Work out the finished part from the listing and answer in its coordinate system (mm). A direction names the side the tool comes from. Coordinates: 2 decimals unless noted, no trailing zeros. Write each loop counter-clockwise with the first axis right and the second up, starting at its lowest first coordinate (ties: lowest second). Pieces come first, ordered by that corner, then holes. Notation, with made-up numbers: (21, 17) - (74, 17) arc R18 ccw to (74, 22) - close; hole circle Ø9 at (28, -31). An arc over 180 degrees is marked (long way). Use one line per item in the form item = value. Start each with the question number.
Item 1: A cutting plane is placed at C-C (y = -12). Write down the section's boundary in (x, z).
Item 2: Consider probe 1 along Y at (x, z) = (1.7, 0); probe 2 along Y at (x, z) = (2.75, 0); probe 3 along X at (y, z) = (-44, -5.5). Determine where each line is inside the solid, lowest interval first.
Item 3: For faces 5 (the cylindrical face through (13.557, 11.892, 0.14)), 6 (the flat face through (10, -39, 0)), determine the directions among +Z, -Z, +X, -X, +Y, -Y from which every point of the face is accessible in a straight line to the end or side of a thin tool.
Item 4: A cutting plane is placed at D-D (y = -71). Write down the section's boundary in (x, z), then the cut area to 3 significant figures.
Item 5: A cutting plane is placed at A-A (z = 0). Write down the section's boundary in (x, y), then the cut area to 3 significant figures.
Item 6: Given pin 1 (2.5 mm diameter, centred on x = 12.5, z = 2, fed in from -Y); pin 2 (1 mm diameter, centred on y = -32.5, z = 0.5, fed in from +X), each flat-ended and moving along its own axis, determine where each tip first touches the part or whether it passes through.
Item 7: A cutting plane is placed at B-B (x = 3). Write down the section's boundary in (y, z), then the cut area to 3 significant figures.
Item 8: Determine the mould class of faces 1 (the flat face through (0, -29, 0)), 2 (the cylindrical face through (2.465, -68.217, 1.774)), 3 (the flat face through (5, -71, 0)), 4 (the flat face through (6, -29, -10)) for opening direction Z: released by +Z, released by -Z, zero draft, split by the parting line, or undercut.
Autodesk Inventor part; units mm, degrees
ref_plane "YZ Plane" through (0, 0, 0) normal (1, 0, 0) x (0, 1, 0)
ref_plane "XZ Plane" through (0, 0, 0) normal (0, 1, 0) x (-1, 0, 0)
ref_plane "XY Plane" through (0, 0, 0) normal (0, 0, 1) x (1, 0, 0)
sketch "스케치1" plane through (0, 0, 0) normal (0, 1, 0) x (-1, 0, 0)
  line L0 (-10, 10) -> (10, 10)
  line L1 (10, 10) -> (10, -10)
  line L2 (10, -10) -> (-10, -10)
  line L3 (-10, -10) -> (-10, 10)
  line L4 (-10, 10) -> (10, -10) construction
  line L5 (10, 10) -> (-10, -10) construction
  line L6 (-10, -10) -> (-15, -10)
  line L7 (-15, -10) -> (-15, 10)
  line L8 (-15, 10) -> (-10, 10)
  line L9 (-10, 10) -> (-10, -10)
  point P0 (0, 0)
  dimension "d0" = 20
  dimension "d1" = 20
  dimension "d2" = 5
extrude "돌출1" add sketch "스케치1" along normal blind 20
extrude "돌출2" add sketch "스케치1" against normal blind 80 contours L0 L1 L2 L3
sketch "스케치2" plane through (-10, 20, -10) normal (-1, 0, 0) x (0, 0, 1)
  line L0 (20, -100) -> (20, 0)
  line L1 (0, 0) -> (20, 0)
  line L2 (0, 0) -> (0, -100)
  line L3 (20, -100) -> (0, -100)
  circle A0 centre (10, -91) radius 3.3
  point P0 (10, -20)
  dimension "d7" = 6.6
  dimension "d8" = 9
sketch "스케치3" plane through (-10, 20, 10) normal (0, 0, 1) x (1, 0, 0)
  line L0 (20, -20) -> (25, -20)
  line L1 (25, -20) -> (25, 0)
  line L2 (0, 0) -> (25, 0)
  line L3 (0, -100) -> (0, 0)
  line L4 (20, -100) -> (0, -100)
  line L5 (20, -20) -> (20, -100)
  line L6 (25, -20) -> (25, 0)
  line L7 (25, 0) -> (0, 0)
  arc A0 (25, -20) -> (20, 0) centre (-10.6945, -18.2986) ccw
  line L8 (20, 0) -> (25, 0)
  line L9 (25, 0) -> (25, -20)
  point P0 (10, -20)
  point P1 (20, 0)
  point P2 (25, -16.5972)
extrude "돌출4" cut sketch "스케치3" against normal blind 20 contours A0 L2 L1
extrude "돌출5" cut sketch "스케치2" against normal blind 10
sketch "스케치4" plane through (-10, -71, 0) normal (-1, 0, 0) x (0, 0, 1)
  circle A0 centre (0, 0) radius 3.3
  point P0 (0, 71)
extrude "돌출6" cut sketch "스케치4" against normal blind 15
sketch "스케치5" plane through (10, 0, 10) normal (0, 0, 1) x (1, 0, 0)
  line L0 (-10, 20) -> (-10, -80)
  line L1 (0, -80) -> (-10, -80)
  line L2 (0, 0) -> (0, -80)
  line L3 (0, 0) -> (5, 0)
  line L4 (5, 0) -> (5, 3.4028)
  arc A0 (5, 3.4028) -> (0, 20) centre (-30.6945, 1.7014) ccw
  line L5 (-10, 20) -> (0, 20)
  circle A1 centre (-5, -12) radius 3
  point P0 (-10, 0)
  dimension "d19" = 6
  dimension "d20" = 32
extrude "돌출7" cut sketch "스케치5" against normal blind 20 contours A1
properties part number "final_탄두조절자ver0.1"
Answer:
q1.outline = (0, -10) - (2, -10) - (2, 10) - (0, 10) - close; (8, -10) - (10, -10) - (10, 10) - (8, 10) - close
q2.probe_1 = -80 to -74.3, -67.7 to 20
q2.probe_2 = -80 to -74.3, -67.7 to -13.98, -10.02 to 20
q2.probe_3 = 0 to 10
q3.face_5 = +Z, -Z, +X, +Y
q3.face_6 = +Z, -Z, +X, -Y
q4.outline = (0, -10) - (10, -10) - (10, 10) - (0, 10) - (0, 3.3) - (5, 3.3) - (5, -3.3) - (0, -3.3) - close
q4.area = 167 mm²
q5.outline = (0, -80) - (10, -80) - (10, 0) - (15, 0) - (15, 3.4) arc R35.73 ccw to (10, 20) - (0, 20) - (0, -67.7) - (5, -67.7) - (5, -74.3) - (0, -74.3) - close; hole circle Ø6 at (5, -12)
q5.area = 1,010 mm²
q6.pin_1 = 0
q6.pin_2 = 10
q7.outline = (-80, -10) - (-14.24, -10) - (-14.24, 10) - (-80, 10) - close; (-9.76, -10) - (20, -10) - (20, 10) - (-9.76, 10) - close; hole circle Ø6.6 at (-71, 0)
q7.area = 1,880 mm²
q8.face_1 = zero draft
q8.face_2 = undercut
q8.face_3 = undercut
q8.face_4 = released by -Z
